from build123d import *

# Parameters (mm, degrees)
F0_W     = 19.051107
F0_H     = 19.05
F0_W_2   = 19.05
F1_DEPTH = 19.05
F2_DEPTH = 38.1
F3_W     = 19.05
F3_H     = 19.05
F4_DEPTH = 19.05


with BuildPart() as f1:
    # F0 (on Top) → F1 (new body)
    with BuildSketch(Plane.XY):
        with Locations((27.630415, 2.113701)):
            Rectangle(F0_W, F0_H)
        with Locations((8.579862, 2.113701)):
            Rectangle(F0_W_2, F0_H)
        with Locations((27.630415, -16.936299)):
            Rectangle(F0_W, F0_H)
    extrude(amount=F1_DEPTH)

    # F0 (on Top) → F2 (join)
    with BuildSketch(Plane.XY):
        with Locations((8.579862, -16.936299)):
            Rectangle(F0_W_2, F0_H)
    extrude(amount=F2_DEPTH)

    # F3 (on face) → F4 (join)
    with BuildSketch(Plane.XZ.offset(26.461299)):
        with Locations((8.579862, 28.575)):
            Rectangle(F3_W, F3_H)
    extrude(amount=F4_DEPTH)


solid = f1.part
Verification items for the finished model (mm, model axes). A direction names the side the tool comes from. Round coordinates to 2 decimals unless told otherwise and drop trailing zeros. Write each loop counter-clockwise with the first axis right and the second up, starting at its lowest first coordinate (ties: lowest second). Pieces come first, ordered by that corner, then holes.
(1) Section check C-C (y = -30). Enter the section's corners in (x, z), plus the area to 3 significant figures.
Returned:
outline: (-0.95, 19.05) - (18.1, 19.05) - (18.1, 38.1) - (-0.95, 38.1) - close
area: 363 mm2
(2) Section check B-B (z = 12). Enter the section's corners in (x, y).
Returned:
outline: (-0.95, -26.46) - (37.16, -26.46) - (37.16, 11.64) - (-0.95, 11.64) - close
(3) Section check A-A (x = 4). Enter the section's corners in (y, z).
Returned:
outline: (-45.51, 19.05) - (-26.46, 19.05) - (-26.46, 0) - (11.64, 0) - (11.64, 19.05) - (-7.41, 19.05) - (-7.41, 38.1) - (-45.51, 38.1) - close
(4) Material ranges on line 1 (Z direction, x = 4.5, y = 5); line 2 (Y direction, x = 23.5, z = 9); line 3 (X direction, y = -42, z = 25.5), recorded low to high.
Returned:
line 1: z = 0 to 19.05
line 2: y = -26.46 to 11.64
line 3: x = -0.95 to 18.1
(5) Depth check by flat-ended pin: pin 1 Ø5.5 at (x, z) = (7.5, 28.5) entering from +Y; pin 2 Ø15 at (y, z) = (-19, 33) entering from +X; pin 3 Ø3 at (x, z) = (27.5, 14) entering from -Y. Enter the tip coordinate at first touch or a pass-through.
Returned:
pin 1: stops at y = -7.41
pin 2: stops at x = 18.1
pin 3: stops at y = -26.46
(6) Access from +Z, -Z, +X, -X, +Y, -Y to the whole of each face (thin tool, end or side, straight path). Record for faces 1 (the flat face through (8, -26, 38.1)), 2 (the flat face through (18.105, -26, 28)), 3 (the flat face through (8, -36, 19.05)), 4 (the flat face through (37.156, -8, 9)), 5 (the flat face through (8, -7.411, 28)).
Returned:
face 1: +Z, +X, -X, +Y, -Y
face 2: +Z, +X, +Y, -Y
face 3: -Z, +X, -X, -Y
face 4: +Z, -Z, +X, +Y, -Y
face 5: +Z, +X, -X, +Y
(7) Section check D-D (y = -9). Enter the section's corners in (x, z), plus the area to 3 significant figures.
Returned:
outline: (-0.95, 0) - (37.16, 0) - (37.16, 19.05) - (18.1, 19.05) - (18.1, 38.1) - (-0.95, 38.1) - close
area: 1,090 mm2
